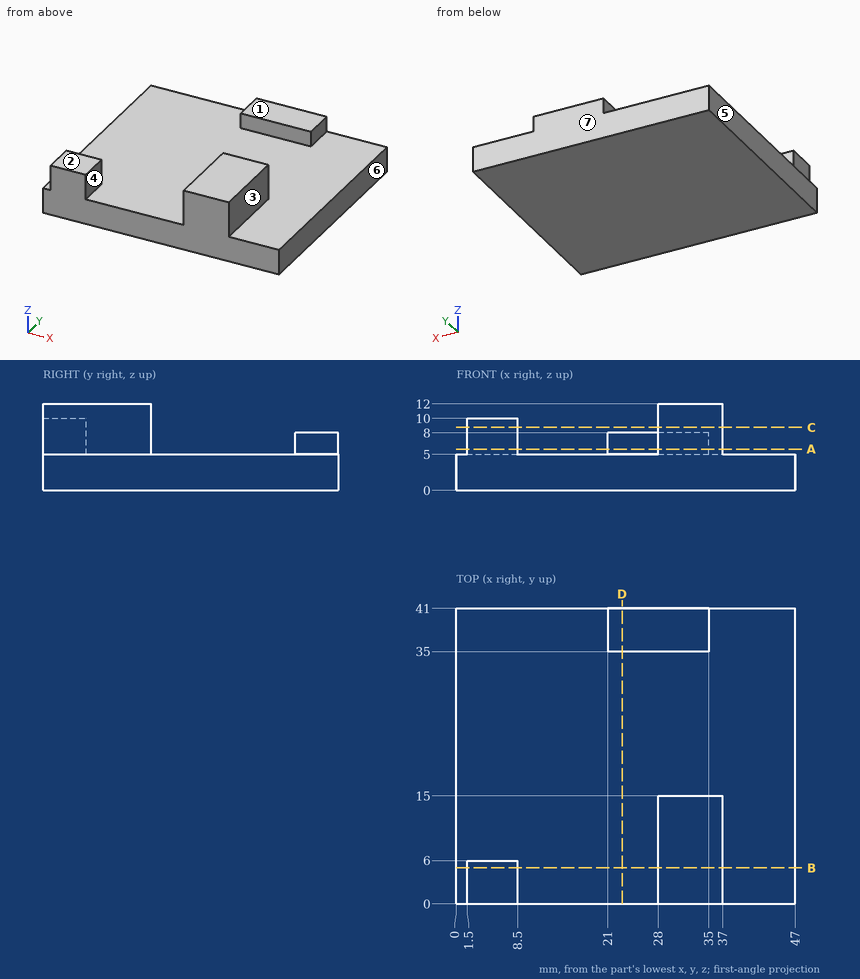
Input: dimensioned drawing with shaded views. Units: mm. Origin: part minimum x, y, z. A direction names the side the tool comes from. Coordinates: 2 decimals unless noted, no trailing zeros. Order: outer loops, then holes, each group sorted by start corner. A loop starts at its lowest first (then second) coordinate and runs counter-clockwise, first axis right, second up. Notation, with made-up numbers: (51, 20) - (77, 20) arc R14 cw to (77, 30) - close; hole circle Ø6 at (42.5, 44.25). An arc over 180 degrees is marked (long way). Return JSON: item names as keys, results as strings. Group by question number.
1. Set-up query: the marked faces 1, 2 and 3. Return all of +Z, -Z, +X, -X, +Y, -Y with unobstructed straight access to the full face (end or side cutting, diameter ignored); none if empty.
2. Cut plane C-C (z = 8.75). Output: boundary loops of the cut face in (x, y), plus the area to 3 significant figures.
3. Material intervals for line 1 along Y through (x, z) = (28.5, 7.5); line 2 along Z through (x, y) = (11, 34); line 3 along Y through (x, z) = (32.5, 9.75), sorted ascending. Write a range as [from, to].
4. Pin query (flat end, axial travel): pin 1 (0.9 mm diameter, centred on y = 39.5, z = 7, fed in from -X); pin 2 (2.5 mm diameter, centred on y = 1.5, z = 8.5, fed in from +X); pin 3 (2 mm diameter, centred on x = 33, z = 9.5, fed in from +Y). Return the tip coordinate at first contact, or that it passes through.
5. Pull-direction query (X, two-part tool) for the marked faces 4, 5, 6 and 7; classes: pulls with the +X half, pulls with the -X half, needs draft (parallel to the pull), parting line crosses it, or undercut.
6. Cut plane A-A (z = 5.75). Output: boundary loops of the cut face in (x, y), plus the area to 3 significant figures.
7. Cut plane D-D (x = 23). Output: boundary loops of the cut face in (y, z), plus the area to 3 significant figures.
8. Cut plane B-B (y = 5). Output: boundary loops of the cut face in (x, z), plus the area to 3 significant figures.
Resolved:
{
 "1": {"face 1": "+Z, +X, -X, +Y", "face 2": "+Z, -X, +Y, -Y", "face 3": "+Z, +X, +Y, -Y"},
 "2": {"outline": "(1.5, 0) - (8.5, 0) - (8.5, 6) - (1.5, 6) - close; (28, 0) - (37, 0) - (37, 15) - (28, 15) - close", "area": "177 mm²"},
 "3": {"line 1": "y = [0, 15], [35, 41]", "line 2": "z = [0, 5]", "line 3": "y = [0, 15]"},
 "4": {"pin 1": "stops at x = 21", "pin 2": "stops at x = 37", "pin 3": "stops at y = 15"},
 "5": {"face 4": "undercut", "face 5": "pulls with the -X half", "face 6": "pulls with the +X half", "face 7": "needs draft"},
 "6": {"outline": "(1.5, 0) - (8.5, 0) - (8.5, 6) - (1.5, 6) - close; (21, 35) - (35, 35) - (35, 41) - (21, 41) - close; (28, 0) - (37, 0) - (37, 15) - (28, 15) - close", "area": "261 mm²"},
 "7": {"outline": "(0, 0) - (41, 0) - (41, 8) - (35, 8) - (35, 5) - (0, 5) - close", "area": "223 mm²"},
 "8": {"outline": "(0, 0) - (47, 0) - (47, 5) - (37, 5) - (37, 12) - (28, 12) - (28, 5) - (8.5, 5) - (8.5, 10) - (1.5, 10) - (1.5, 5) - (0, 5) - close", "area": "333 mm²"}
}
